Check sheet for the modelled part. Datum: model origin and axes. Units: mm. Face numbers are marked on the shaded views. Give positions to 0.01 mm unless a question says otherwise; leave off trailing zeros. Write each loop counter-clockwise with the first axis right and the second up, starting at its lowest first coordinate (ties: lowest second). Pieces come first, ordered by that corner, then holes. Notation, with made-up numbers: (43.25, 54.25) -> (51.25, 54.25) arc R27 cw to (51.25, 86.25) -> close; hole circle Ø10 at (-4.5, 39). An arc over 180 degrees is marked (long way). Answer as a JSON object with one key per item and string values.
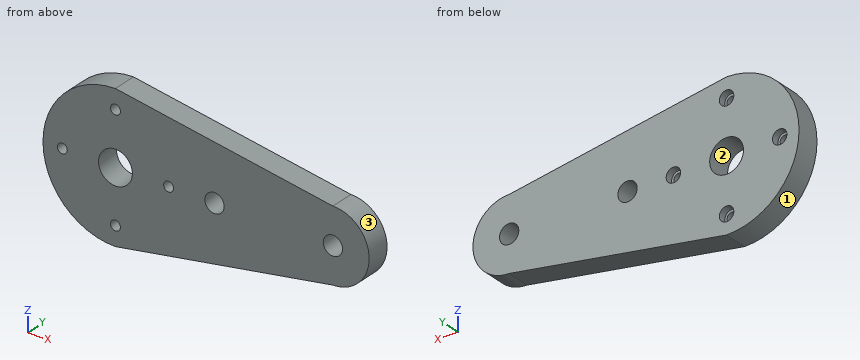
Autodesk Inventor part; units mm, degrees
ref_plane "YZ Plane" through (0, 0, 0) normal (1, 0, 0) x (0, 1, 0)
ref_plane "XZ Plane" through (0, 0, 0) normal (0, 1, 0) x (-1, 0, 0)
ref_plane "XY Plane" through (0, 0, 0) normal (0, 0, 1) x (1, 0, 0)
sketch "Sketch1" plane through (0, 0, 0) normal (0, 1, 0) x (-1, 0, 0)
  circle A0 centre (0, 0) radius 22
  line L0 (0, 0) -> (0, -22)
  circle A1 centre (0, -22) radius 1.55
  circle A2 centre (0, -22) radius 3
  circle A3 centre (22, 0) radius 3
  circle A4 centre (22, 0) radius 1.55
  circle A5 centre (0, 22) radius 3
  circle A6 centre (0, 22) radius 1.55
  circle A7 centre (-22, 0) radius 3
  circle A8 centre (-22, 0) radius 1.55
  circle A9 centre (0, 0) radius 30
  line L1 (0, 0) -> (-90, 0)
  circle A10 centre (-90, 0) radius 4
  circle A11 centre (-90, 0) radius 15
  line L2 (0, -30) -> (-90, -15)
  line L3 (0, 30) -> (-90, 15)
  circle A12 centre (0, 0) radius 5
  dimension "d0" = 44
  dimension "d1" = 3.1
  dimension "d2" = 6
  dimension "d5" = 360
  dimension "d7" = 60
  dimension "d8" = 90
  dimension "d9" = 8
  dimension "d10" = 30
  dimension "d11" = 10
extrude "Extrusion1" add sketch "Sketch1" along normal blind 10 contours A0 A4 | A0 A4 | A4 A0 A3 | A0 A3 A4 | A3 A0 A2 L0 A12 L1 A7 A5 | A9 L3 L2 | A9 L2 A11 L1 | L1 A11 L3 A9 | A5 A0 A6 | A0 A6 A5 | A2 A0 A1 | A0 A1 L0 A2 | A6 A0 | A0 A6 | A1 A0 | A0 L0 A1 | A2 A0 A7 L1 A12 L0 | L0 A1 A0 A2 | A7 L1 A8 A0 | A0 A8 L1 A7 | A0 A1 L0 | A12 L1 L0 | L0 L1 A12 | A8 L1 A0 | A0 L1 A8 | A7 A0 A8 L1 | L1 A8 A0 A7 | L1 A8 A0 | A0 A8 L1 | A11
sketch "Sketch2" plane through (0, 0, 0) normal (0, -1, 0) x (1, 0, 0)
  circle A0 centre (0, 22) radius 1.5
  circle A1 centre (0, -22) radius 1.5
  circle A2 centre (22, 0) radius 1.5
  circle A3 centre (-22, 0) radius 1.5
  circle A4 centre (0, 22) radius 2.05
  circle A5 centre (22, 0) radius 2.05
  circle A6 centre (-22, 0) radius 2.05
  circle A7 centre (0, -22) radius 2.05
  circle A8 centre (-22, 0) radius 2.05
  circle A9 centre (0, 22) radius 2.05
  circle A10 centre (22, 0) radius 2.05
  circle A11 centre (0, -22) radius 2.05
  point P0 (0, 0)
  dimension "d16" = 3
  dimension "d17" = 3
  dimension "d19" = 3
  dimension "d21" = 3
  dimension "d34" = 4.1
  dimension "d35" = 4.1
  dimension "d36" = 4.1
  dimension "d37" = 4.1
  dimension "d38" = 4.1
  dimension "d39" = 4.1
  dimension "d40" = 4.1
  dimension "d41" = 4.1
extrude "Extrusion2" cut sketch "Sketch2" against normal blind 10 contours A0 | A1 | A2 | A3
sketch "Sketch3" plane through (0, 10, 0) normal (0, 1, 0) x (1, 0, 0)
  circle A0 centre (0, -22) radius 1.5
  line L0 (0, 0) -> (0, -22)
  circle A1 centre (-22, 0) radius 1.5
  line L1 (0, 0) -> (-22, 0)
  circle A2 centre (0, 22) radius 1.5
  line L2 (0, 0) -> (0, 22)
  circle A3 centre (22, 0) radius 1.5
  line L3 (0, 0) -> (22, 0)
  circle A4 centre (0, -22) radius 3
  circle A5 centre (22, 0) radius 3
  circle A6 centre (0, 22) radius 3
  circle A7 centre (-22, 0) radius 3
  dimension "d24" = 6
  dimension "d27" = 360
extrude "Extrusion3" cut sketch "Sketch3" against normal blind 3
sketch "Sketch4" plane through (0, 0, 0) normal (0, -1, 0) x (1, 0, 0)
  circle A0 centre (0, 0) radius 5
  circle A1 centre (0, 0) radius 7
  point P0 (0, 0)
  dimension "d31" = 14
extrude "Extrusion4" cut sketch "Sketch4" against normal blind 2.5
ref_plane "Work Plane1" through (0, 0, 0) normal (0, -1, 0) x (1, 0, 0)
sketch "Sketch5" plane through (0, 0, 0) normal (0, -1, 0) x (1, 0, 0)
  circle A0 centre (0, 22) radius 1.5
  circle A1 centre (0, 22) radius 2.05
  circle A2 centre (-22, 0) radius 2.05
  circle A3 centre (0, -22) radius 2.05
  circle A4 centre (22, 0) radius 2.05
  point P0 (0, 0)
  dimension "d43" = 4.1
  dimension "d46" = 360
extrude "Extrusion5" cut sketch "Sketch5" against normal blind 10
sketch "Sketch6" plane through (0, 0, 0) normal (0, -1, 0) x (1, 0, 0)
  circle A0 centre (0, 0) radius 7
extrude "Extrusion6" cut sketch "Sketch6" against normal blind 70.5
sketch "Sketch7" plane through (0, 0, 0) normal (0, -1, 0) x (1, 0, 0)
  circle A0 centre (90, 0) radius 4
  circle A1 centre (41, 0) radius 4
  point P0 (0, 0)
  dimension "d53" = 8
extrude "Extrusion7" cut sketch "Sketch7" against normal blind 29.5 contours A1
properties part number "motormount"
1. Sectioned sample at A-A, the plane y = 5. Enter the section's corners in (x, z).
Determined:
{"outline": "(0, -30) -> (90, -15) arc R15 ccw to (90, 15) -> (0, 30) arc R30 ccw to start; hole circle Ø4.1 at (-22, 0); hole circle Ø14 at (0, 0); hole circle Ø4.1 at (0, -22); hole circle Ø4.1 at (0, 22); hole circle Ø4.1 at (22, 0); hole circle Ø8 at (41, 0); hole circle Ø8 at (90, 0)"}
2. Sectioned sample at D-D, the plane x = 66. Enter the section's corners in (y, z), plus the area to 3 significant figures.
Determined:
{"outline": "(0, -19) -> (10, -19) -> (10, 19) -> (0, 19) -> close", "area": "380 mm^2"}
3. Go/stop test with flat-tipped pins: P1, Ø1.5, axis at y = 5, z = -5.5, coming from the +X side; P2, Ø5, axis at x = -6, y = 5, coming from the +Z side; P3, Ø1.8, axis at x = -1, z = -23.5, coming from the +Y side. Record where each tip stops, or that it passes through.
Determined:
{"P1": "x = 104.23", "P2": "z = 29.8", "P3": "y = 7"}
4. Mould release check, pull along X, two halves, no side actions. Record for the marked faces 1, 2 and 3: released by +X, released by -X, zero draft, split by the parting line, or undercut.
Determined:
{"face 1": "released by -X", "face 2": "undercut", "face 3": "released by +X"}
5. Sectioned sample at B-B, the plane z = 22. Enter the section's corners in (x, y), plus the area to 3 significant figures.
Determined:
{"outline": "(-20.4, 0) -> (-2.05, 0) -> (-2.05, 7) -> (-3, 7) -> (-3, 10) -> (-20.4, 10) -> close; (2.05, 0) -> (48, 0) -> (48, 10) -> (3, 10) -> (3, 7) -> (2.05, 7) -> close", "area": "637 mm^2"}
6. Sectioned sample at C-C, the plane x = 41.5. Enter the section's corners in (y, z).
Determined:
{"outline": "(0, -23.08) -> (10, -23.08) -> (10, -3.97) -> (0, -3.97) -> close; (0, 3.97) -> (10, 3.97) -> (10, 23.08) -> (0, 23.08) -> close"}
7. Scan lines: L1, parallel to Z at x = 0, y = 5.25; L2, parallel to Y at x = 2, z = 20.5; L3, parallel to Z at x = -22, y = 8.45. Record each from-to range of solid material in increasing order. Write a range as [from, to].
Determined:
{"L1": "[-30, -24.05], [-19.95, -7], [7, 19.95], [24.05, 30]", "L2": "[0, 7]", "L3": "[-20.4, -3], [3, 20.4]"}
